The model under review builds one solid part; all positions refer to its coordinate system, in mm. Round coordinates to 2 decimals unless told otherwise and drop trailing zeros. Loops run counter-clockwise (first coordinate to the right, second up) from the corner with the lowest first, then second, coordinate; pieces in that order, holes last. Notation, with made-up numbers: M 85.5,-6 L 137.5,-6 A9 ccw 137.5,4 Z; hole C -10,50.5 d9. An arc over 180 degrees is marked long. Answer in a Markdown table with one row per item. Add a question column.
from build123d import *

# Parameters (mm, degrees)
F0_R     = 2.38125
F1_DEPTH = 0.79375
F2_R     = 0.508
F3_R     = 0.508


with BuildPart() as f1:
    # F0 (on Front) → F1 (new body, symmetric)
    with BuildSketch(Plane.XZ):
        Polygon((0.7529974873, 5.447464528), (-4.3411439238, 3.375847217), (-5.0941414111, -2.071617311), (-0.7529974873, -5.447464528), (4.3411439238, -3.375847217), (5.0941414111, 2.071617311), align=None)
        Circle(F0_R, mode=Mode.SUBTRACT)
    extrude(amount=F1_DEPTH, both=True)

    # F2
    f2_edges = [f1.edges().sort_by_distance(p)[0] for p in [
        (-2.38125, -0.79375, 0),
    ]]
    fillet(f2_edges, radius=F2_R)

    # F3
    f3_edges = [f1.edges().sort_by_distance(p)[0] for p in [
        (-2.38125, 0.79375, 0),
    ]]
    fillet(f3_edges, radius=F3_R)


solid = f1.part
1. To check wall thickness, follow probe 1 along Z at (x, y) = (0, -0.2); probe 2 along X at (y, z) = (-0.05, 0.25); probe 3 along X at (y, z) = (-0.5, -0.75). State the ranges of each line that lie inside material, in increasing order.
2. Take a section at B-B, the plane z = 0. State the section outline as (x, y) points.
3. Take a section at D-D, the plane z = 4.75. State the section outline as (x, y) points, and give its area (3 significant figures).
4. Take a section at C-C, the plane x = -3.75. State the section outline as (y, z) points.
5. Take a section at A-A, the plane x = 0. State the section outline as (y, z) points.
6. For pin 1 Ø3 at (x, z) = (0, 0) entering from +Y, flat-tipped, find the tip position at first contact; note if it passes through.
Check sheet entries:
| question | item | result |
|---|---|---|
| 1 | probe 1 | z = -5.14 to -2.38, 2.38 to 5.14 |
| 1 | probe 2 | x = -4.77 to -2.37, 2.37 to 4.84 |
| 1 | probe 3 | x = -4.91 to -2.31, 2.31 to 4.7 |
| 2 | outline | M -4.81,-0.79 L -2.89,-0.79 A0.51 ccw -2.38,-0.29 L -2.38,0.29 A0.51 ccw -2.89,0.79 L -4.81,0.79 Z; M 2.38,-0.29 A0.51 ccw 2.89,-0.79 L 4.81,-0.79 L 4.81,0.79 L 2.89,0.79 A0.51 ccw 2.38,0.29 Z |
| 3 | outline | M -0.96,-0.79 L 1.65,-0.79 L 1.65,0.79 L -0.96,0.79 Z |
| 3 | area | 4.15 mm^2 |
| 4 | outline | M -0.79,-3.12 L 0.79,-3.12 L 0.79,3.62 L -0.79,3.62 Z |
| 5 | outline | M -0.79,-5.14 L 0.79,-5.14 L 0.79,-2.89 A0.51 ccw 0.29,-2.38 L -0.29,-2.38 A0.51 ccw -0.79,-2.89 Z; M -0.79,2.89 A0.51 ccw -0.29,2.38 L 0.29,2.38 A0.51 ccw 0.79,2.89 L 0.79,5.14 L -0.79,5.14 Z |
| 6 | pin 1 | passes through |
